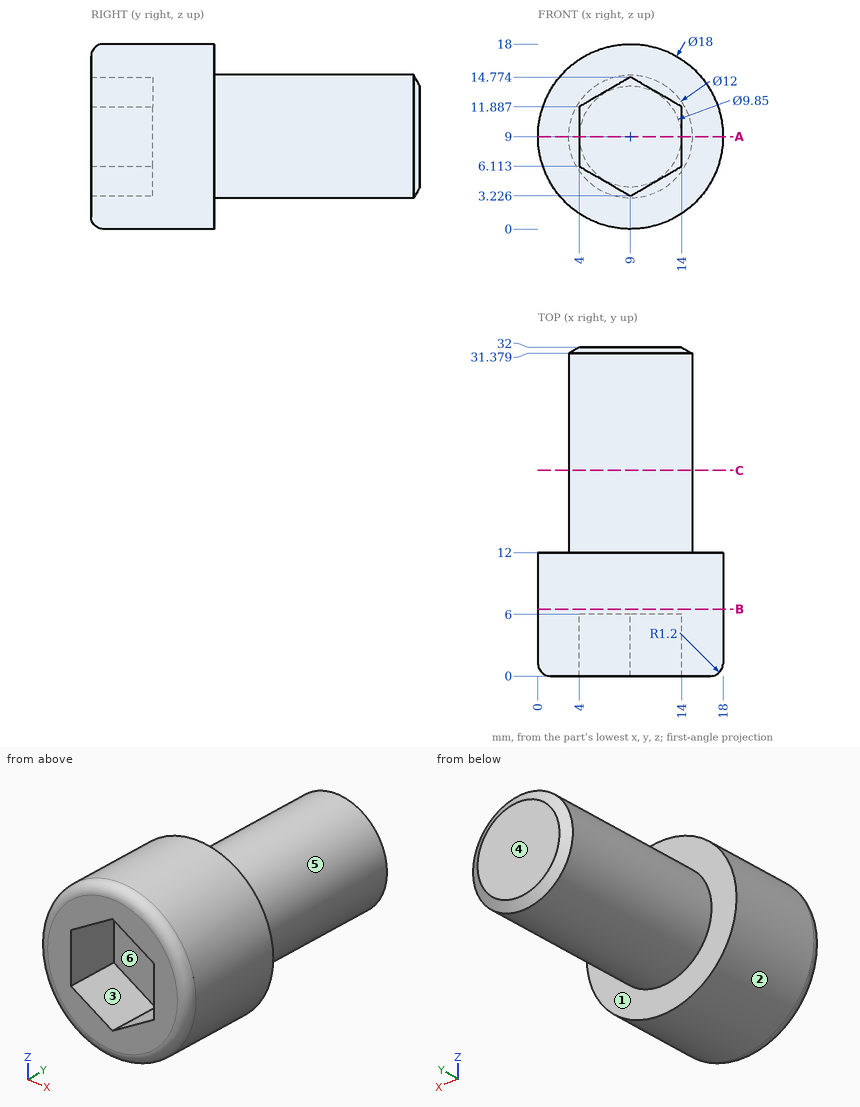
Design review of the part shown in the three views and the two pictorial views. Dimensions are in mm from the part's minimum x, y and z. A direction names the side the tool comes from. Round coordinates to 2 decimals unless told otherwise and drop trailing zeros. Write each loop counter-clockwise with the first axis right and the second up, starting at its lowest first coordinate (ties: lowest second). Pieces come first, ordered by that corner, then holes. Notation, with made-up numbers: M 60,-18 L 82,-18 A14 cw 82,-10 Z; hole C 38,-8 d8. An arc over 180 degrees is marked long. Use a Markdown table: item, result. Add a question column.
Q1. To check wall thickness, follow line 1 (Y direction, x = 12.5, z = 11); line 2 (Y direction, x = 13.5, z = 14.75); line 3 (X direction, y = 5.5, z = 5.25) (1 decimal). State the ranges of each line that lie inside material, in increasing order.
Q2. We need section A-A, the plane z = 9. State the section outline as (x, y) points (1 decimal), plus the area to 3 significant figures.
Q3. Insertion check: pin 1 (1.5 mm diameter, centred on y = 26, z = 12, fed in from +X); pin 2 (4 mm diameter, centred on y = 28, z = 11, fed in from +X); pin 3 (4 mm diameter, centred on x = 7.5, y = 27, fed in from -Z). Each pin has a flat end and moves straight along its axis. Give the tip position at first contact, or say it passes through.
Q4. We need section B-B, the plane y = 6.5. State the section outline as (x, z) points.
Q5. We need section C-C, the plane y = 20. State the section outline as (x, z) points, plus the area to 3 significant figures.
Q6. Machinability: for the marked faces 4, 5 and 6, which of the approach directions +Z, -Z, +X, -X, +Y, -Y give a long, thin tool a straight path to every point of the face, cutting with its end or side? Answer none if there is none.
Q7. The part is to be moulded in two halves that separate along X. For the marked faces 1, 2 and 3, say which applies: pulls with the +X half, pulls with the -X half, needs draft (parallel to the pull), parting line crosses it, or undercut.
Findings below:
| question | item | result |
|---|---|---|
| 1 | line 1 | y = 6 to 32 |
| 1 | line 2 | y = 0 to 12 |
| 1 | line 3 | x = 0.8 to 5.5, 12.5 to 17.2 |
| 2 | outline | M 0,1.2 A1.2 ccw 1.2,0 L 4,0 L 4,6 L 14,6 L 14,0 L 16.8,0 A1.2 ccw 18,1.2 L 18,12 L 15,12 L 15,31.4 L 13.9,32 L 4.1,32 L 3,31.4 L 3,12 L 0,12 Z |
| 2 | area | 395 mm² |
| 3 | pin 1 | stops at x = 14.56 |
| 3 | pin 2 | stops at x = 15 |
| 3 | pin 3 | stops at z = 3 |
| 4 | outline | C 9,9 d18 |
| 5 | outline | C 9,9 d12 |
| 5 | area | 113 mm² |
| 6 | face 4 | +Z, -Z, +X, -X, +Y |
| 6 | face 5 | +Y |
| 6 | face 6 | -Y |
| 7 | face 1 | needs draft |
| 7 | face 2 | parting line crosses it |
| 7 | face 3 | undercut |
